```python
from build123d import *

# Parameters (mm, degrees)
SKETCH1_W           = 42
SKETCH1_H           = 18
BOSS_EXTRUDE1_DEPTH = 3
SKETCH2_W           = 11
SKETCH2_H           = 3
BOSS_EXTRUDE2_DEPTH = 9
SKETCH3_R           = 2.5
CUT_EXTRUDE1_DEPTH  = 47.572524089
SKETCH4_W           = 15
SKETCH4_H           = 12
CUT_EXTRUDE2_DEPTH  = 3
FILLET1_R           = 2
FILLET2_R           = 2


with BuildPart() as part:
    # Sketch1 → Boss-Extrude1 (new body)
    with BuildSketch(Plane(origin=(0, 0, 0), x_dir=(1, 0, 0), z_dir=(0, 1, 0))):
        with Locations((21, 9)):
            Rectangle(SKETCH1_W, SKETCH1_H)
    extrude(amount=BOSS_EXTRUDE1_DEPTH)

    # Sketch2 → Boss-Extrude2 (add)
    with BuildSketch(Plane.XZ):
        with Locations((36.5, -1.5)):
            Rectangle(SKETCH2_W, SKETCH2_H)
        with Locations((36.5, -16.5)):
            Rectangle(SKETCH2_W, SKETCH2_H)
    extrude(amount=BOSS_EXTRUDE2_DEPTH)

    # Sketch3 → Cut-Extrude1 (cut, through all)
    with BuildSketch(Plane.XY):
        with Locations((36.5, -4.5)):
            Circle(SKETCH3_R)
    extrude(amount=-CUT_EXTRUDE1_DEPTH, mode=Mode.SUBTRACT)

    # Sketch4 → Cut-Extrude2 (cut)
    with BuildSketch(Plane(origin=(0, 3, 0), x_dir=(1, 0, 0), z_dir=(0, 1, 0))):
        with Locations((34.5, 9)):
            Rectangle(SKETCH4_W, SKETCH4_H)
    extrude(amount=-CUT_EXTRUDE2_DEPTH, mode=Mode.SUBTRACT)

    # Fillet1
    fillet1_edges = [part.edges().sort_by_distance(p)[0] for p in [
        (0, 1.5, -18),
        (0, 1.5, 0),
    ]]
    fillet(fillet1_edges, radius=FILLET1_R)

    # Fillet2
    fillet2_edges = [part.edges().sort_by_distance(p)[0] for p in [
        (42, 3, -1.5),
        (42, -9, -1.5),
        (31, -9, -1.5),
        (42, -9, -16.5),
        (31, -9, -16.5),
        (42, 3, -16.5),
    ]]
    fillet(fillet2_edges, radius=FILLET2_R)


solid = part.part
```
Can you work these out from the model? Positions are in its coordinate system, mm. A direction names the side the tool comes from. Round coordinates to 2 decimals unless told otherwise and drop trailing zeros. Loops run counter-clockwise (first coordinate to the right, second up) from the corner with the lowest first, then second, coordinate; pieces in that order, holes last. Notation, with made-up numbers: M 53.5,-17 L 69.5,-17 A21 cw 69.5,10 Z; hole C 30.25,86.25 d9. An arc over 180 degrees is marked long. Answer as a JSON object with one key per item and string values. Group by question number.
Q1. Imagine slicing it at B-B, the plane x = 36.5. Please give me the cut outline in (y, z).
Q2. Will these pins go through, and if not, where does the flat tip stop? pin 1 (4.5 mm diameter, centred on x = 36.5, y = -4.5, fed in from +Z); pin 2 (1.5 mm diameter, centred on y = -3, z = -16.5, fed in from -X); pin 3 (2.5 mm diameter, centred on y = 1, z = -7, fed in from +X); pin 4 (8 mm diameter, centred on x = 8, z = -3, fed in from -Y).
Q3. Imagine slicing it at C-C, the plane y = -4.5. Please give me the cut outline in (x, z), then the cut area to 3 significant figures.
Q4. Imagine slicing it at D-D, the plane x = 28.5. Please give me the cut outline in (y, z).
Q5. Imagine slicing it at A-A, the plane y = -1. Please give me the cut outline in (x, z).
Q6. On a 3-axis mill with a long thin cutter (end or side, diameter ignored), from which of +Z, -Z, +X, -X, +Y, -Y can I reach the whole of each face in a straight line? I mean faces 1 (the flat face through (31, -3, -17)), 2 (the flat face through (27, 2, -9)), 3 (the flat face through (26, 1, 0)). Say none if no direction works.
Q7. We'd pull the mould along X, two halves only. Please class faces 4 (the flat face through (28, 1, -18)), 5 (the cylindrical face through (0.57, 1.52, -0.6)), 6 (the cylindrical face through (38.81, -5.46, -16.48)): +X half, -X half, draft (parallel to the pull), parting line (faces both ways), or undercut.
Q8. Please list where these lines run through material, in increasing order: L1, parallel to Y at x = 36.5, z = -1.3; L2, parallel to Z at x = 30, y = 0.75; L3, parallel to X at y = 0.25, z = -12.25.
Findings:
{
 "1": {"outline": "M -9,-18 L -7,-18 L -7,-15 L -9,-15 Z; M -9,-3 L -7,-3 L -7,0 L -9,0 Z; M -2,-18 L 3,-18 L 3,-15 L -2,-15 Z; M -2,-3 L 3,-3 L 3,0 L -2,0 Z"},
 "2": {"pin 1": "passes through", "pin 2": "stops at x = 31", "pin 3": "stops at x = 27", "pin 4": "stops at y = 0"},
 "3": {"outline": "M 31,-18 L 34,-18 L 34,-15 L 31,-15 Z; M 31,-3 L 34,-3 L 34,0 L 31,0 Z; M 39,-18 L 42,-18 L 42,-15 L 39,-15 Z; M 39,-3 L 42,-3 L 42,0 L 39,0 Z", "area": "36.0 mm2"},
 "4": {"outline": "M 0,-18 L 3,-18 L 3,-15 L 0,-15 Z; M 0,-3 L 3,-3 L 3,0 L 0,0 Z"},
 "5": {"outline": "M 31,-18 L 42,-18 L 42,-15 L 31,-15 Z; M 31,-3 L 42,-3 L 42,0 L 31,0 Z"},
 "6": {"face 1": "+Z, -Z, -X, -Y", "face 2": "+X, +Y, -Y", "face 3": "+Z, +X, -X, +Y, -Y"},
 "7": {"face 4": "draft", "face 5": "-X half", "face 6": "undercut"},
 "8": {"L1": "y = -9 to -7, -2 to 3", "L2": "z = -18 to -15, -3 to 0", "L3": "x = 0 to 27"}
}
